Source: CAD feature listing. Evaluate the final solid. Frame: model axes, mm. Round coordinates to 2 decimals unless told otherwise and drop trailing zeros. Write each loop counter-clockwise with the first axis right and the second up, starting at its lowest first coordinate (ties: lowest second). Pieces come first, ordered by that corner, then holes. Notation, with made-up numbers: (56, 39) -> (77, 39) arc R28 cw to (77, 67) -> close; hole circle Ø6 at (26.25, -14.5). An arc over 180 degrees is marked (long way). Put each result on its own line as item: value.
```python
from build123d import *

# Parameters (mm, degrees)
F2_DEPTH = 5.08
F1_R     = 1.905
F3_DEPTH = 12.7


with BuildPart() as f2:
    # F0 (on Top) → F2 (new body)
    with BuildSketch(Plane.XY):
        Polygon((89.55228, 53.388856), (-26.639517, 53.388856), (-64.403486, 53.388856), (-69.483486, 53.388856), (-69.483486, 48.308856), (-69.483486, -49.658944), (-69.483486, -54.738944), (-64.403486, -54.738944), (-26.639517, -54.738944), (89.55228, -54.738944), (94.63228, -54.738944), (94.63228, 12.150785), (94.63228, 53.388856), align=None)
    extrude(amount=-F2_DEPTH)

    # F1 (on Top) → F3 (join)
    with BuildSketch(Plane.XY):
        with Locations((-66.943486, -52.198944)):
            Circle(F1_R)
        with Locations((-66.943486, 50.848856)):
            Circle(F1_R)
        with Locations((92.09228, 50.848856)):
            Circle(F1_R)
        with Locations((92.09228, -52.198944)):
            Circle(F1_R)
    extrude(amount=F3_DEPTH)


solid = f2.part
```
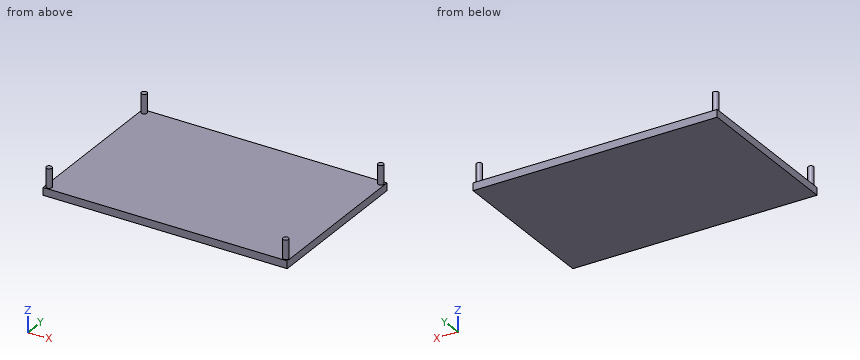
Q1. Cut plane C-C on z = 3. Output: boundary loops of the cut face in (x, y) (3 decimals), and give its area (3 significant figures).
Ans:
outline: circle Ø3.81 at (-66.943, -52.199); circle Ø3.81 at (-66.943, 50.849); circle Ø3.81 at (92.092, -52.199); circle Ø3.81 at (92.092, 50.849)
area: 45.6 mm^2
Q2. Material intervals for line 1 (Z direction, x = -11.5, y = 35.5), sorted ascending. Write a range as [from, to].
Ans:
line 1: z = [-5.08, 0]
Q3. Pin query (flat end, axial travel): pin 1 (1.5 mm diameter, centred on x = 65, y = -29.5, fed in from +Z); pin 2 (3 mm diameter, centred on x = 67, z = 3, fed in from -Y). Return the tip coordinate at first contact, or that it passes through.
Ans:
pin 1: stops at z = 0
pin 2: passes through
Q4. Cut plane A-A on y = 23.5. Output: boundary loops of the cut face in (x, z).
Ans:
outline: (-69.48, -5.08) -> (94.63, -5.08) -> (94.63, 0) -> (-69.48, 0) -> close
Q5. Cut plane B-B on x = 44.5. Output: boundary loops of the cut face in (y, z).
Ans:
outline: (-54.74, -5.08) -> (53.39, -5.08) -> (53.39, 0) -> (-54.74, 0) -> close
